The listing builds one solid part. Answer for the finished solid, in the listing's coordinates (mm). Face numbers are marked on the shaded views. A direction names the side the tool comes from. Round coordinates to 2 decimals unless told otherwise and drop trailing zeros. Write each loop counter-clockwise with the first axis right and the second up, starting at its lowest first coordinate (ties: lowest second). Pieces come first, ordered by that corner, then holes.
from build123d import *

# Parameters (mm, degrees)
SKETCH_4_W           = 46
SKETCH_4_H           = 107.5
EXTRUDE_1_DEPTH      = 3
SKETCH_5_W           = 23.5
SKETCH_5_H           = 56
EXTRUDE_2_DEPTH      = 12.4
SKETCH_6_R           = 0.75
CUT_EXTRUDE_1_DEPTH  = 66.1949768
SKETCH_6_5_R         = 1.5
CUT_EXTRUDE_4_DEPTH  = 1.2
CUT_EXTRUDE_START    = -22.3
SKETCH_6_6_R         = 1.5
CUT_EXTRUDE_5_DEPTH  = 1.2
SKETCH_7_R           = 0.7
CUT_EXTRUDE_6_DEPTH  = 2
SKETCH_9_W           = 46
SKETCH_9_H           = 8
EXTRUDE_3_DEPTH      = 3
SKETCH_10_R          = 0.6
CUT_EXTRUDE_8_DEPTH  = 2
CUT_EXTRUDE_START_2  = -105.5
SKETCH_10_2_R        = 0.6
CUT_EXTRUDE_9_DEPTH  = 2
SKETCH_11_R          = 0.6
CUT_EXTRUDE_10_DEPTH = 2
SKETCH_12_W          = 44
SKETCH_12_H          = 12.4
CUT_EXTRUDE_11_DEPTH = 0.5
CUT_EXTRUDE_START_3  = -23.5
SKETCH_12_2_W        = 44
SKETCH_12_2_H        = 12.4
CUT_EXTRUDE_12_DEPTH = 0.5
SKETCH_13_R          = 0.6
CUT_EXTRUDE_13_DEPTH = 2
CUT_EXTRUDE_START_4  = -44
SKETCH_13_2_R        = 0.6
CUT_EXTRUDE_14_DEPTH = 2
SKETCH_14_R          = 5.05
CUT_EXTRUDE_15_DEPTH = 2


with BuildPart() as part:
    # 草图4 → 凸台-拉伸1 (new body)
    with BuildSketch(Plane(origin=(0, 0, 0), x_dir=(1, 0, 0), z_dir=(0, 1, 0))):
        Rectangle(SKETCH_4_W, SKETCH_4_H)
    extrude(amount=EXTRUDE_1_DEPTH)

    # 草图5 → 凸台-拉伸2 (add)
    with BuildSketch(Plane.XZ):
        Rectangle(SKETCH_5_W, SKETCH_5_H)
    extrude(amount=EXTRUDE_2_DEPTH)

    # 草图6 → 切除-拉伸1 (cut, through all)
    with BuildSketch(Plane.ZY.offset(11.75)):
        with Locations((25, -12.4)):
            Circle(SKETCH_6_R)
        with Locations((-25, -12.4)):
            Circle(SKETCH_6_R)
    extrude(amount=-CUT_EXTRUDE_1_DEPTH, mode=Mode.SUBTRACT)

    # 草图6<5> → 切除-拉伸4 (cut)
    with BuildSketch(Plane.ZY.offset(11.75)):
        with Locations((25, -12.4)):
            Circle(SKETCH_6_5_R)
        with Locations((-25, -12.4)):
            Circle(SKETCH_6_5_R)
    extrude(amount=-CUT_EXTRUDE_4_DEPTH, mode=Mode.SUBTRACT)

    # 草图6<6> → 切除-拉伸5 (cut)
    with BuildSketch(Plane.ZY.offset(11.75).offset(CUT_EXTRUDE_START)):
        with Locations((25, -12.4)):
            Circle(SKETCH_6_6_R)
        with Locations((-25, -12.4)):
            Circle(SKETCH_6_6_R)
    extrude(amount=-CUT_EXTRUDE_5_DEPTH, mode=Mode.SUBTRACT)

    # 草图7 → 切除-拉伸6 (cut)
    with BuildSketch(Plane(origin=(0, -12.4, 0), x_dir=(-1, 0, 0), z_dir=(0, -1, 0))):
        with Locations(Location((9.249949764, -20, 0), (0, 0, 90))):
            Circle(SKETCH_7_R)
        with Locations(Location((-9.249949764, -20, 0), (0, 0, 90))):
            Circle(SKETCH_7_R)
        with Locations(Location((-9.249949764, -6, 0), (0, 0, 90))):
            Circle(SKETCH_7_R)
        with Locations(Location((9.249949764, -6, 0), (0, 0, 90))):
            Circle(SKETCH_7_R)
        with Locations(Location((9.249949764, 6, 0), (0, 0, 90))):
            Circle(SKETCH_7_R)
        with Locations(Location((-9.249949764, 6, 0), (0, 0, 90))):
            Circle(SKETCH_7_R)
        with Locations(Location((-9.249949764, 20, 0), (0, 0, 90))):
            Circle(SKETCH_7_R)
        with Locations(Location((9.249949764, 20, 0), (0, 0, 90))):
            Circle(SKETCH_7_R)
    extrude(amount=-CUT_EXTRUDE_6_DEPTH, mode=Mode.SUBTRACT)

    # 草图9 → 凸台-拉伸3 (add)
    with BuildSketch(Plane.XZ):
        with Locations((0, 49.75)):
            Rectangle(SKETCH_9_W, SKETCH_9_H)
        with Locations((0, -49.75)):
            Rectangle(SKETCH_9_W, SKETCH_9_H)
    extrude(amount=EXTRUDE_3_DEPTH)

    # 草图10 → 切除-拉伸8 (cut)
    with BuildSketch(Plane.XY.offset(53.75)):
        with Locations((-7.5, 0)):
            Circle(SKETCH_10_R)
        with Locations((7.5, 0)):
            Circle(SKETCH_10_R)
    extrude(amount=-CUT_EXTRUDE_8_DEPTH, mode=Mode.SUBTRACT)

    # 草图10<2> → 切除-拉伸9 (cut)
    with BuildSketch(Plane.XY.offset(53.75).offset(CUT_EXTRUDE_START_2)):
        with Locations((-7.5, 0)):
            Circle(SKETCH_10_2_R)
        with Locations((7.5, 0)):
            Circle(SKETCH_10_2_R)
    extrude(amount=-CUT_EXTRUDE_9_DEPTH, mode=Mode.SUBTRACT)

    # 草图11 → 切除-拉伸10 (cut)
    with BuildSketch(Plane(origin=(0, 3, 0), x_dir=(1, 0, 0), z_dir=(0, 1, 0))):
        with Locations(Location((-18.1, 30, 0), (0, 0, 270))):
            Circle(SKETCH_11_R)
        with Locations(Location((18.1, 30, 0), (0, 0, 270))):
            Circle(SKETCH_11_R)
        with Locations(Location((18.1, -30, 0), (0, 0, 270))):
            Circle(SKETCH_11_R)
        with Locations(Location((-18.1, -30, 0), (0, 0, 270))):
            Circle(SKETCH_11_R)
    extrude(amount=-CUT_EXTRUDE_10_DEPTH, mode=Mode.SUBTRACT)

    # 草图12 → 切除-拉伸11 (cut)
    with BuildSketch(Plane.ZY.offset(11.75)):
        with Locations((0, -6.2)):
            Rectangle(SKETCH_12_W, SKETCH_12_H)
    extrude(amount=-CUT_EXTRUDE_11_DEPTH, mode=Mode.SUBTRACT)

    # 草图12<2> → 切除-拉伸12 (cut)
    with BuildSketch(Plane.ZY.offset(11.75).offset(CUT_EXTRUDE_START_3)):
        with Locations((0, -6.2)):
            Rectangle(SKETCH_12_2_W, SKETCH_12_2_H)
    extrude(amount=CUT_EXTRUDE_12_DEPTH, mode=Mode.SUBTRACT)

    # 草图13 → 切除-拉伸13 (cut)
    with BuildSketch(Plane(origin=(23, 0, 0), x_dir=(0, 0, -1), z_dir=(1, 0, 0))):
        with Locations((-30, 1.5)):
            Circle(SKETCH_13_R)
        with Locations((30, 1.5)):
            Circle(SKETCH_13_R)
    extrude(amount=-CUT_EXTRUDE_13_DEPTH, mode=Mode.SUBTRACT)

    # 草图13<2> → 切除-拉伸14 (cut)
    with BuildSketch(Plane(origin=(23, 0, 0), x_dir=(0, 0, -1), z_dir=(1, 0, 0)).offset(CUT_EXTRUDE_START_4)):
        with Locations((-30, 1.5)):
            Circle(SKETCH_13_2_R)
        with Locations((30, 1.5)):
            Circle(SKETCH_13_2_R)
    extrude(amount=-CUT_EXTRUDE_14_DEPTH, mode=Mode.SUBTRACT)

    # 草图14 → 切除-拉伸15 (cut)
    with BuildSketch(Plane(origin=(0, 3, 0), x_dir=(1, 0, 0), z_dir=(0, 1, 0))):
        with Locations(Location((-12, 22.5, 0), (0, 0, 270))):
            Circle(SKETCH_14_R)
        with Locations(Location((12, 22.5, 0), (0, 0, 270))):
            Circle(SKETCH_14_R)
        with Locations(Location((-12, -22.5, 0), (0, 0, 270))):
            Circle(SKETCH_14_R)
        with Locations(Location((12, -22.5, 0), (0, 0, 270))):
            Circle(SKETCH_14_R)
    extrude(amount=-CUT_EXTRUDE_15_DEPTH, mode=Mode.SUBTRACT)


solid = part.part
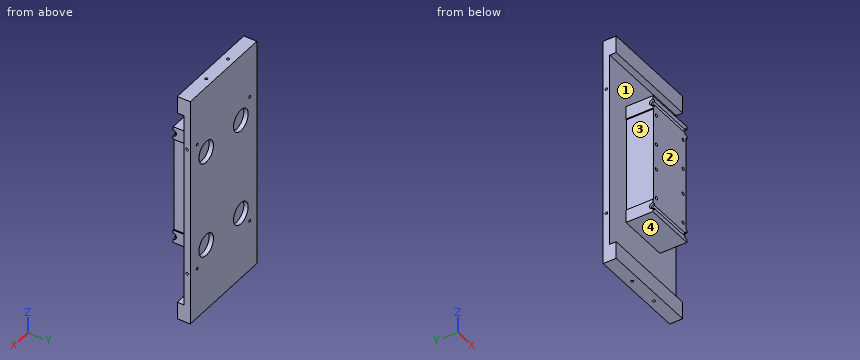
1. Straight lines are drawn through the part: line 1 along X through (y, z) = (1.7, -22.5); line 2 along X through (y, z) = (-11.9, 20); line 3 along Z through (x, y) = (9.5, -2). For each, find the intervals that lie inside material, in ascending order.
Geometry says:
line 1: x = -23 to -17.05, -6.95 to 6.95, 17.05 to 23
line 2: x = -11.25 to -9.95, -8.55 to 8.55, 9.95 to 11.25
line 3: z = -53.75 to -45.75, -28 to 28, 45.75 to 53.75
2. Given pin 1 (0.7 mm diameter, centred on y = 1.5, z = 30, fed in from +X); pin 2 (0.7 mm diameter, centred on x = 9.5, z = 20, fed in from -Y); pin 3 (1 mm diameter, centred on x = 6.5, y = -6.5, fed in from +Z), each flat-ended and moving along its own axis, determine where each tip first touches the part or whether it passes through.
Geometry says:
pin 1: stops at x = 21
pin 2: stops at y = -10.4
pin 3: stops at z = 28
3. Section C-C on y = -9 is taken. Determine the outline of the cut face in (x, z).
Geometry says:
outline: (-11.75, -28) - (11.75, -28) - (11.75, -22) - (11.25, -22) - (11.25, 22) - (11.75, 22) - (11.75, 28) - (-11.75, 28) - (-11.75, 22) - (-11.25, 22) - (-11.25, -22) - (-11.75, -22) - close
4. A tool of negligible diameter and unlimited length cuts with its end or side. For the marked faces 1, 2, 3 and 4, from which of +Z, -Z, +X, -X, +Y, -Y can it reach the whole face along a straight path? Write none if from no direction.
Geometry says:
face 1: -Y
face 2: +Z, -Z, +X, -X, -Y
face 3: -X, -Y
face 4: +X, -X, -Y
5. Section D-D on x = -16 is taken. Determine the outline of the cut face in (y, z), plus the area to 3 significant figures.
Geometry says:
outline: (-3, -53.75) - (3, -53.75) - (3, -25.58) - (1, -25.58) - (1, -19.42) - (3, -19.42) - (3, 19.42) - (1, 19.42) - (1, 25.58) - (3, 25.58) - (3, 53.75) - (-3, 53.75) - (-3, 45.75) - (0, 45.75) - (0, -45.75) - (-3, -45.75) - close
area: 346 mm2
6. Section B-B on z = -9 is taken. Determine the outline of the cut face in (x, y).
Geometry says:
outline: (-23, 0) - (-11.25, 0) - (-11.25, -12.4) - (11.25, -12.4) - (11.25, 0) - (23, 0) - (23, 3) - (-23, 3) - close
7. Section A-A on y = -2 is taken. Determine the outline of the cut face in (x, z).
Geometry says:
outline: (-23, -53.75) - (23, -53.75) - (23, -45.75) - (-23, -45.75) - close; (-23, 45.75) - (23, 45.75) - (23, 53.75) - (-23, 53.75) - close; (-11.75, -28) - (11.75, -28) - (11.75, -22) - (11.25, -22) - (11.25, 22) - (11.75, 22) - (11.75, 28) - (-11.75, 28) - (-11.75, 22) - (-11.25, 22) - (-11.25, -22) - (-11.75, -22) - close
